Source: three-view drawing plus pictorial views. Frame: mm from the lowest corner of the part. A direction names the side the tool comes from. Give positions to 0.01 mm unless a question says otherwise; leave off trailing zeros. Order: outer loops, then holes, each group sorted by start corner. A loop starts at its lowest first (then second) coordinate and runs counter-clockwise, first axis right, second up. Notation, with made-up numbers: M 28.5,36.25 L 72.5,36.25 A15 cw 72.5,60.25 Z; hole C 20,-31.75 d10. An arc over 180 degrees is marked long. One line per item, written item: value. Start each with the question number.
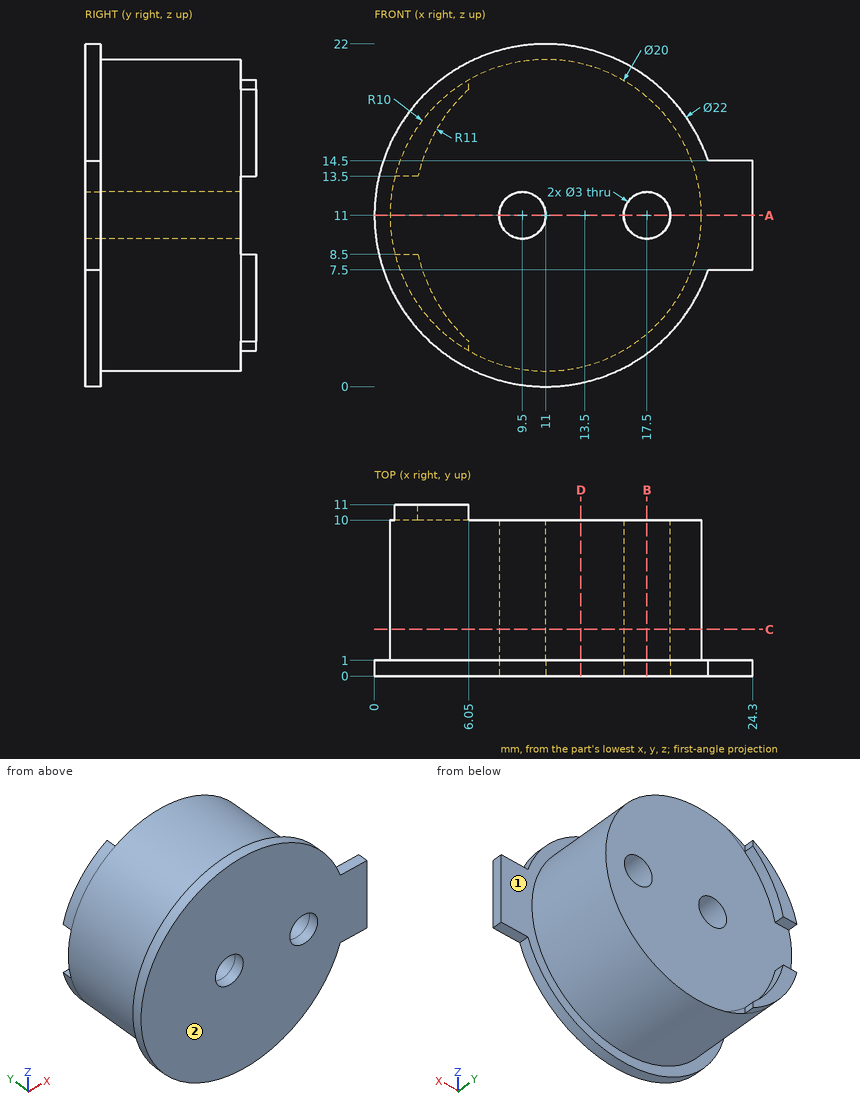
Q1. Contact query for flat-ended pins moving along their axis: pin 1 (0.7 mm diameter, centred on x = 6.5, z = 19.5, fed in from +Y); pin 2 (0.8 mm diameter, centred on x = 23.5, y = 0.5, fed in from -Z); pin 3 (0.5 mm diameter, centred on x = 2, y = 10.5, fed in from -Z); pin 4 (1.8 mm diameter, centred on x = 9.5, z = 11, fed in from -Y). Output: stop coordinate, or through.
Q2. Section query D-D on x = 13.25. Return loops of the section in (y, z).
Q3. Section query C-C on y = 3. Return loops of the section in (x, z).
Q4. Section query B-B on x = 17.5. Return loops of the section in (y, z), and give its area (3 significant figures).
Q5. Ray query, line 1 along X through (y, z) = (4.5, 11); line 2 along X through (y, z) = (9, 11.75); line 3 along Z through (x, y) = (17.5, 0.3). Return the intervals inside material, ascending. Write a range as [from, to].
Q6. Section query A-A on z = 11. Return loops of the section in (x, y), and give its area (3 significant figures).
Q7. Set-up query: the marked faces 1 and 2. Return all of +Z, -Z, +X, -X, +Y, -Y with unobstructed straight access to the full face (end or side cutting, diameter ignored); none if empty.
Results below:
1. pin 1: y = 10
1. pin 2: z = 7.5
1. pin 3: z = 6.16
1. pin 4: through
2. outline: M 0,0.23 L 1,0.23 L 1,1.26 L 10,1.26 L 10,20.74 L 1,20.74 L 1,21.77 L 0,21.77 Z
3. outline: C 11,11 d20; hole C 9.5,11 d3; hole C 17.5,11 d3
4. outline: M 0,2.13 L 1,2.13 L 1,3.4 L 10,3.4 L 10,9.5 L 0,9.5 Z; M 0,12.5 L 10,12.5 L 10,18.6 L 1,18.6 L 1,19.87 L 0,19.87 Z
4. area: 125 mm2
5. line 1: [1, 8], [11, 16], [19, 21]
5. line 2: [1.03, 8.2], [10.8, 16.2], [18.8, 20.97]
5. line 3: [2.13, 9.5], [12.5, 19.87]
6. outline: M 0,0 L 8,0 L 8,10 L 1,10 L 1,1 L 0,1 Z; M 11,0 L 16,0 L 16,10 L 11,10 Z; M 19,0 L 24.3,0 L 24.3,1 L 21,1 L 21,10 L 19,10 Z
6. area: 144 mm2
7. face 1: +Y
7. face 2: +Z, -Z, +X, -X, -Y
